from build123d import *

# Parameters (mm, degrees)
SKIZZE1_W                       = 300
SKIZZE1_H                       = 75
LINEAR_AUSTRAGEN1_DEPTH         = 10
SKIZZE2_W                       = 100
SKIZZE2_H                       = 60
SCHNITT_LINEAR_AUSTRAGEN1_DEPTH = 10
VERRUNDUNG1_R                   = 3


with BuildPart() as part:
    # Skizze1 → Linear austragen1 (new body)
    with BuildSketch(Plane.XY):
        with Locations((0, -112.5)):
            Rectangle(SKIZZE1_W, SKIZZE1_H)
    extrude(amount=LINEAR_AUSTRAGEN1_DEPTH)

    # Skizze2 → Schnitt-Linear austragen1 (cut)
    with BuildSketch(Plane.XY.offset(10)):
        with Locations((0, -110)):
            Rectangle(SKIZZE2_W, SKIZZE2_H)
    extrude(amount=-SCHNITT_LINEAR_AUSTRAGEN1_DEPTH, mode=Mode.SUBTRACT)

    # Verrundung1
    verrundung1_edges = [part.edges().sort_by_distance(p)[0] for p in [
        (50, -80, 5),
        (50, -140, 5),
        (-50, -140, 5),
        (-50, -80, 5),
    ]]
    fillet(verrundung1_edges, radius=VERRUNDUNG1_R)


solid = part.part
Model file for the job. Use its own axes, mm. A direction names the side the tool comes from. Give positions to 0.01 mm unless a question says otherwise; leave off trailing zeros. Loops run counter-clockwise (first coordinate to the right, second up) from the corner with the lowest first, then second, coordinate; pieces in that order, holes last.
1) Saw through at A-A (x = -28). Write the cut outline in (y, z), plus the area to 3 significant figures.
2) Saw through at C-C (y = -134). Write the cut outline in (x, z), plus the area to 3 significant figures.
3) Tool access for faces 4 (the flat face through (-150, -113, 5)), 5 (the flat face through (-1, -140, 5)): list every direction of +Z, -Z, +X, -X, +Y, -Y with a clear straight run to the whole face (end or side of a thin tool).
4) Wall check: line 1 (Y direction, x = -33.5, z = 1); line 2 (X direction, y = -132, z = 4.5); line 3 (X direction, y = -138.5, z = 5.75). Give the ranges that are in metal, low to high.
5) Pull direction X, two halves, no side cores. Call faces 1 (the flat face through (150, -113, 5)), 2 (the flat face through (-2, -75, 5)), 3 (the flat face through (-50, -110, 5)): +X half, -X half, draft (parallel to the pull), parting line (faces both ways), or undercut.
6) Saw through at B-B (z = 8). Write the cut outline in (x, y).
Answer block:
1. outline: (-150, 0) - (-140, 0) - (-140, 10) - (-150, 10) - close; (-80, 0) - (-75, 0) - (-75, 10) - (-80, 10) - close
1. area: 150 mm2
2. outline: (-150, 0) - (-50, 0) - (-50, 10) - (-150, 10) - close; (50, 0) - (150, 0) - (150, 10) - (50, 10) - close
2. area: 2,000 mm2
3. face 4: +Z, -Z, -X, +Y, -Y
3. face 5: +Z, -Z
4. line 1: y = -150 to -140, -80 to -75
4. line 2: x = -150 to -50, 50 to 150
4. line 3: x = -150 to -49.6, 49.6 to 150
5. face 1: +X half
5. face 2: draft
5. face 3: undercut
6. outline: (-150, -150) - (150, -150) - (150, -75) - (-150, -75) - close; hole (-50, -137) arc R3 ccw to (-47, -140) - (47, -140) arc R3 ccw to (50, -137) - (50, -83) arc R3 ccw to (47, -80) - (-47, -80) arc R3 ccw to (-50, -83) - close
